Source: three-view drawing plus pictorial views. Frame: mm from the lowest corner of the part. A direction names the side the tool comes from. Round coordinates to 2 decimals unless told otherwise and drop trailing zeros. Loops run counter-clockwise (first coordinate to the right, second up) from the corner with the lowest first, then second, coordinate; pieces in that order, holes last. Notation, with made-up numbers: M 20,44.5 L 76,44.5 A6 cw 76,52.5 Z; hole C 65.5,-8.75 d7. An arc over 180 degrees is marked long. Answer as a JSON object with one key per item and string values.
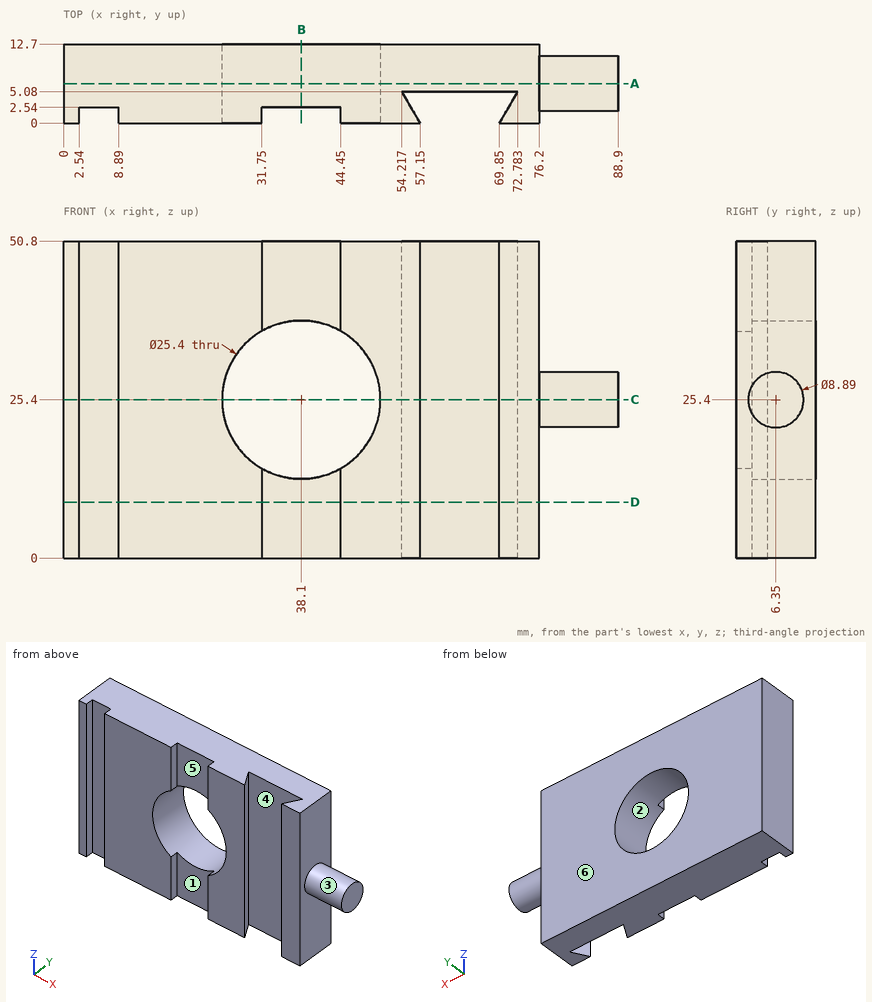
1) Cut plane C-C on z = 25.4. Return the cut outline in (x, y) (3 decimals).
Geometry results:
{"outline": "M 0,0 L 2.54,0 L 2.54,2.54 L 8.89,2.54 L 8.89,0 L 25.4,0 L 25.4,12.7 L 0,12.7 Z; M 50.8,0 L 57.15,0 L 54.217,5.08 L 72.783,5.08 L 69.85,0 L 76.2,0 L 76.2,1.905 L 88.9,1.905 L 88.9,10.795 L 76.2,10.795 L 76.2,12.7 L 50.8,12.7 Z"}
2) Cut plane D-D on z = 9. Return the cut outline in (x, y).
Geometry results:
{"outline": "M 0,0 L 2.54,0 L 2.54,2.54 L 8.89,2.54 L 8.89,0 L 31.75,0 L 31.75,2.54 L 44.45,2.54 L 44.45,0 L 57.15,0 L 54.22,5.08 L 72.78,5.08 L 69.85,0 L 76.2,0 L 76.2,12.7 L 0,12.7 Z"}
3) Cut plane A-A on y = 6.35. Return the cut outline in (x, z) (3 decimals).
Geometry results:
{"outline": "M 0,0 L 76.2,0 L 76.2,20.955 L 88.9,20.955 L 88.9,29.845 L 76.2,29.845 L 76.2,50.8 L 0,50.8 Z; hole C 38.1,25.4 d25.4"}
4) Cut plane B-B on x = 38.1. Return the cut outline in (y, z), and give its area (3 significant figures).
Geometry results:
{"outline": "M 2.54,0 L 12.7,0 L 12.7,12.7 L 2.54,12.7 Z; M 2.54,38.1 L 12.7,38.1 L 12.7,50.8 L 2.54,50.8 Z", "area": "258 mm2"}
5) First-contact query: pin 1 (4 mm diameter, centred on y = 4.5, z = 13, fed in from +X); pin 2 (5 mm diameter, centred on y = 10, z = 21, fed in from +X); pin 3 (5.5 mm diameter, centred on x = 65.5, z = 30.5, fed in from -Y); pin 4 (3 mm diameter, centred on x = 5.5, z = 18.5, fed in from -Y). Flat tips, straight axial feed; report the tip coordinate or a pass-through.
Geometry results:
{"pin 1": "x = 76.2", "pin 2": "x = 88.9", "pin 3": "y = 5.08", "pin 4": "y = 2.54"}
6) Pull-direction query (Y, two-part tool) for the marked faces 1, 2, 3 and 4; classes: +Y half, -Y half, draft (parallel to the pull), parting line (faces both ways), or undercut.
Geometry results:
{"face 1": "-Y half", "face 2": "draft", "face 3": "parting line", "face 4": "undercut"}
7) Line query: probe 1 along Z at (x, y) = (38.1, 8.25); probe 2 along X at (y, z) = (5.75, 25.4); probe 3 along X at (y, z) = (2.5, 25.4). Output: solid intervals per line, ascending.
Geometry results:
{"probe 1": "0 to 12.7, 38.1 to 50.8", "probe 2": "0 to 25.4, 50.8 to 88.9", "probe 3": "0 to 2.54, 8.89 to 25.4, 50.8 to 55.71, 71.29 to 88.9"}
8) Set-up query: the marked faces 5 and 6. Return all of +Z, -Z, +X, -X, +Y, -Y with unobstructed straight access to the full face (end or side cutting, diameter ignored); none if empty.
Geometry results:
{"face 5": "+Z, -Z, -Y", "face 6": "+Z, -Z, +X, -X, +Y"}
